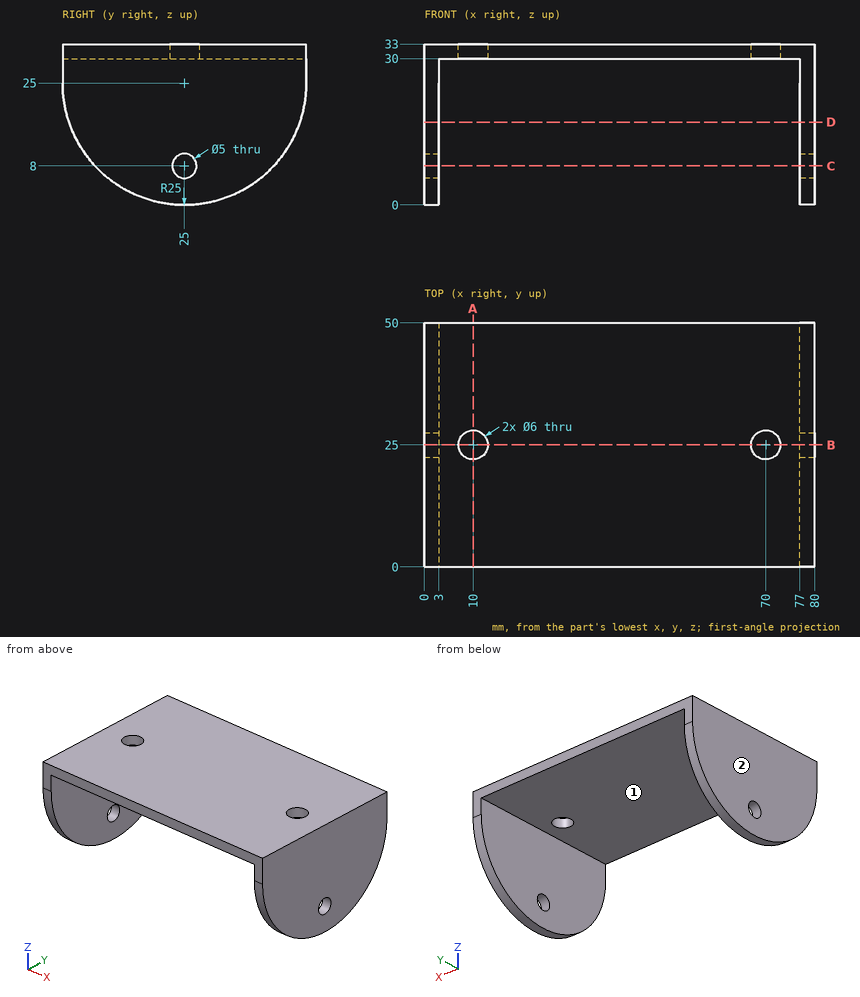
Geometry: see drawing. Coordinates: mm, zero at the bounding-box minimum. A direction names the side the tool comes from. Give positions to 0.01 mm unless a question says otherwise; leave off trailing zeros. Order: outer loops, then holes, each group sorted by start corner. A loop starts at its lowest first (then second) coordinate and runs counter-clockwise, first axis right, second up.
1. Line query: probe 1 along X at (y, z) = (31, 3.5); probe 2 along Y at (x, z) = (10, 32); probe 3 along Z at (x, y) = (4, 25.5). Output: solid intervals per line, ascending.
Computed:
probe 1: x = 0 to 3, 77 to 80
probe 2: y = 0 to 22, 28 to 50
probe 3: z = 30 to 33
2. Cut plane C-C (z = 8). Return loops of the section in (x, y).
Computed:
outline: (0, 6.67) - (3, 6.67) - (3, 22.5) - (0, 22.5) - close; (0, 27.5) - (3, 27.5) - (3, 43.33) - (0, 43.33) - close; (77, 6.67) - (80, 6.67) - (80, 22.5) - (77, 22.5) - close; (77, 27.5) - (80, 27.5) - (80, 43.33) - (77, 43.33) - close
3. Cut plane B-B (y = 25). Return loops of the section in (x, z).
Computed:
outline: (0, 0) - (3, 0) - (3, 5.5) - (0, 5.5) - close; (0, 10.5) - (3, 10.5) - (3, 30) - (7, 30) - (7, 33) - (0, 33) - close; (13, 30) - (67, 30) - (67, 33) - (13, 33) - close; (73, 30) - (77, 30) - (77, 10.5) - (80, 10.5) - (80, 33) - (73, 33) - close; (77, 0) - (80, 0) - (80, 5.5) - (77, 5.5) - close
4. Pin query (flat end, axial travel): pin 1 Ø25 at (x, y) = (22.5, 27.5) entering from -Z; pin 2 Ø4 at (y, z) = (25, 8) entering from +X. Return the tip coordinate at first contact, or that it passes through.
Computed:
pin 1: stops at z = 30
pin 2: passes through
5. Cut plane D-D (z = 17). Return loops of the section in (x, y).
Computed:
outline: (0, 1.31) - (3, 1.31) - (3, 48.69) - (0, 48.69) - close; (77, 1.31) - (80, 1.31) - (80, 48.69) - (77, 48.69) - close
6. Set-up query: the marked faces 1 and 2. Return all of +Z, -Z, +X, -X, +Y, -Y with unobstructed straight access to the full face (end or side cutting, diameter ignored); none if empty.
Computed:
face 1: -Z, +Y, -Y
face 2: +Z, -Z, -X, +Y, -Y
7. Cut plane A-A (x = 10). Return loops of the section in (y, z).
Computed:
outline: (0, 30) - (22, 30) - (22, 33) - (0, 33) - close; (28, 30) - (50, 30) - (50, 33) - (28, 33) - close
